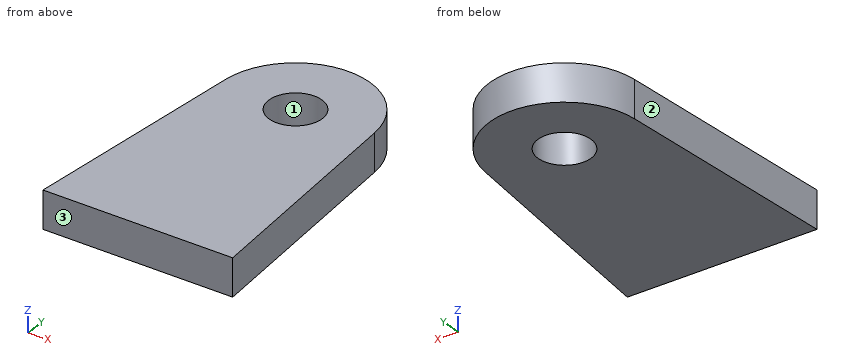
from build123d import *

# Parameters (mm, degrees)
BOSS_EXTRUDE1_DEPTH      = 3.175
M4_CLEARANCE_HOLE1_D     = 4.5
M4_CLEARANCE_HOLE1_DEPTH = 16.002
M4_CLEARANCE_HOLE1_TIP   = 1.351936393


with BuildPart() as part:
    # Sketch1 → Boss-Extrude1 (new body)
    with BuildSketch(Plane.XY):
        with BuildLine():
            Line((0, 0), (16.081830017, 0))
            Line((16.081830017, 0), (14.366751341, 19.603438966))
            ThreePointArc((14.366751341, 19.603438966), (8.040915009, 25.4), (1.715078676, 19.603438966))
            Line((1.715078676, 19.603438966), (0, 0))
        make_face()
    extrude(amount=BOSS_EXTRUDE1_DEPTH)

    # M4 Clearance Hole1
    with Locations(Plane.XY.offset(3.175)):
        with Locations((8.040915009, 19.05)):
            Hole(M4_CLEARANCE_HOLE1_D / 2, depth=M4_CLEARANCE_HOLE1_DEPTH)
            with Locations((0, 0, -(M4_CLEARANCE_HOLE1_DEPTH + M4_CLEARANCE_HOLE1_TIP / 2))):  # 118° drill point
                Cone(0, M4_CLEARANCE_HOLE1_D / 2, M4_CLEARANCE_HOLE1_TIP, mode=Mode.SUBTRACT)


solid = part.part
Read the model definition and answer for the solid it produces. Units are mm, in the model's axes. Face numbers are marked on the shaded views. Round coordinates to 2 decimals unless told otherwise and drop trailing zeros. Loops run counter-clockwise (first coordinate to the right, second up) from the corner with the lowest first, then second, coordinate; pieces in that order, holes last.
Q1. Section D-D on y = 6.25 is taken. Write down the section's boundary in (x, z) (3 decimals).
Q2. Consider probe 1 along X at (y, z) = (20.25, 2.65); probe 2 along Y at (x, z) = (7.25, 2.3); probe 3 along Y at (x, z) = (13.75, 0.75). Determine where each line is inside the solid, lowest interval first.
Q3. Determine the mould class of the marked faces 1, 2 and 3 for opening direction Y: released by +Y, released by -Y, zero draft, split by the parting line, or undercut.
Q4. Section A-A on x = 9.75 is taken. Write down the section's boundary in (y, z) (3 decimals).
Q5. Each of these flat-tipped pins is pushed along its axis until it touches: pin 1 (1 mm diameter, centred on x = 9.5, z = 0.5, fed in from +Y); pin 2 (3.5 mm diameter, centred on x = 8.04, y = 19.05, fed in from +Z). Where does it stop, or does it pass through?
Q6. Section C-C on z = 1.7 is taken. Write down the section's boundary in (x, y), and give its area (3 significant figures).
Q7. Section B-B on y = 19.05 is taken. Write down the section's boundary in (x, z) (3 decimals), and give its area (3 significant figures).
Output:
1. outline: (0.547, 0) - (15.535, 0) - (15.535, 3.175) - (0.547, 3.175) - close
2. probe 1: x = 1.81 to 6.14, 9.94 to 14.28
2. probe 2: y = 0 to 16.94, 21.16 to 25.35
2. probe 3: y = 0 to 21.83
3. face 1: undercut
3. face 2: released by +Y
3. face 3: released by -Y
4. outline: (0, 0) - (17.587, 0) - (17.587, 3.175) - (0, 3.175) - close; (20.513, 0) - (25.166, 0) - (25.166, 3.175) - (20.513, 3.175) - close
5. pin 1: stops at y = 25.33
5. pin 2: passes through
6. outline: (0, 0) - (16.08, 0) - (14.37, 19.6) arc R6.35 ccw to (1.72, 19.6) - close; hole circle Ø4.5 at (8.04, 19.05)
6. area: 322 mm2
7. outline: (1.667, 0) - (5.791, 0) - (5.791, 3.175) - (1.667, 3.175) - close; (10.291, 0) - (14.415, 0) - (14.415, 3.175) - (10.291, 3.175) - close
7. area: 26.2 mm2
